```python
from build123d import *

# Parameters (mm, degrees)
F0_W     = 50.8
F0_H     = 101.6
F0_W_2   = 44.45
F0_H_2   = 95.25
F1_DEPTH = 1670.05
F3_DEPTH = 228.6
F4_R     = 5.08


with BuildPart() as f1:
    # F0 (on Front) → F1 (new body)
    with BuildSketch(Plane.XZ):
        with Locations((25.4, 50.8)):
            Rectangle(F0_W, F0_H)
        with Locations((25.4, 50.8)):
            Rectangle(F0_W_2, F0_H_2, mode=Mode.SUBTRACT)
    extrude(amount=F1_DEPTH)

    # F2 (on face) → F3 (cut)
    with BuildSketch(Plane.XY.offset(101.6)):
        Polygon((50.8, -1619.25), (0, -1670.05), (50.8, -1670.05), align=None)
        Polygon((50.8, 0), (0, 0), (50.8, -50.8), align=None)
    extrude(amount=-F3_DEPTH, mode=Mode.SUBTRACT)

    # F4
    f4_edges = [f1.edges().sort_by_distance(p)[0] for p in [
        (50.8, -835.025, 101.6),
        (50.8, -835.025, 0),
        (0, -835.025, 101.6),
        (0, -835.025, 0),
    ]]
    fillet(f4_edges, radius=F4_R)


solid = f1.part
```
Could you check a few things on this model? Use its own coordinates, in mm. A direction names the side the tool comes from. Round coordinates to 2 decimals unless told otherwise and drop trailing zeros. Loops run counter-clockwise (first coordinate to the right, second up) from the corner with the lowest first, then second, coordinate; pieces in that order, holes last.
Q1. I want a section at B-B (z = 46). Write out the boundary of the cut face in (x, y) (3 decimals).
Q2. I want a section at C-C (y = -1135.5). Write out the boundary of the cut face in (x, z) (3 decimals), and give its area (3 significant figures).
Q3. For P1, Ø8, axis at x = 6, z = 39, coming from the +Y side, with a flat end and sliding along its axis, tell me the tip position at first contact or that it passes through.
Q4. Please list where these lines run through material, in increasing order: L1, parallel to Z at x = 18, y = -1231 (3 decimals); L2, parallel to X at y = -1039.5, z = 29.5 (3 decimals); L3, parallel to Z at x = 3.5, y = -228 (3 decimals).
Q5. I want a section at A-A (x = 35). Write out the boundary of the cut face in (y, z) (3 decimals), and give its area (3 significant figures).
Q6. On a 3-axis mill with a long thin cutter (end or side, diameter ignored), from which of +Z, -Z, +X, -X, +Y, -Y can I reach the whole of each face in a straight line? I mean faces 1 (the flat face through (47.625, -824, 50)), 2 (the flat face through (25, -823, 0)). Say none if no direction works.
Answer below:
1. outline: (0, -1670.05) - (3.175, -1666.875) - (3.175, -3.175) - (0, 0) - close; (47.625, -1622.425) - (50.8, -1619.25) - (50.8, -50.8) - (47.625, -47.625) - close
2. outline: (0, 5.08) arc R5.08 ccw to (5.08, 0) - (45.72, 0) arc R5.08 ccw to (50.8, 5.08) - (50.8, 96.52) arc R5.08 ccw to (45.72, 101.6) - (5.08, 101.6) arc R5.08 ccw to (0, 96.52) - close; hole (3.175, 3.175) - (47.625, 3.175) - (47.625, 98.425) - (3.175, 98.425) - close
2. area: 905 mm2
3. P1: stops at y = -2
4. L1: z = 0 to 3.175, 98.425 to 101.6
4. L2: x = 0 to 3.175, 47.625 to 50.8
4. L3: z = 0.252 to 3.175, 98.425 to 101.348
5. outline: (-1635.05, 0) - (-35, 0) - (-35, 3.175) - (-1635.05, 3.175) - close; (-1635.05, 98.425) - (-35, 98.425) - (-35, 101.6) - (-1635.05, 101.6) - close
5. area: 10,200 mm2
6. face 1: +Y, -Y
6. face 2: -Z, +X, -X, +Y, -Y
